CAD build for the part. Positions are in the model's coordinates, mm. Face numbers are marked on the shaded views. A direction names the side the tool comes from. Give positions to 0.01 mm unless a question says otherwise; leave off trailing zeros. Loops run counter-clockwise (first coordinate to the right, second up) from the corner with the lowest first, then second, coordinate; pieces in that order, holes last. Notation, with made-up numbers: (87.25, 28.25) -> (118.25, 28.25) arc R20 cw to (118.25, 47.25) -> close; hole circle Ø8 at (20, 20). An arc over 180 degrees is marked (long way). Use one line per item in the form item = value.
```python
from build123d import *

# Parameters (mm, degrees)
SKETCH_R        = 1.8
PAD_DEPTH       = 5
POCKET_DEPTH    = 2.3800001144
POCKET001_DEPTH = 1
SKETCH003_R     = 3
POCKET002_DEPTH = 3


with BuildPart() as part:
    # Sketch → Pad (new body)
    with BuildSketch(Plane.XY):
        with BuildLine():
            ThreePointArc((-7, -13.2664991614), (7.7459666924, -12.8452325787), (15, 0))
            Line((15, 30), (15, 0))
            ThreePointArc((15, 30), (7.7459666924, 42.8452325787), (-7, 43.2664991614))
            Line((-7, 43.2664991614), (-7, -13.2664991614))
        make_face()
        with Locations((0, 30)):
            Circle(SKETCH_R, mode=Mode.SUBTRACT)
        Circle(SKETCH_R, mode=Mode.SUBTRACT)
    extrude(amount=PAD_DEPTH)

    # Sketch001 → Pocket (cut)
    with BuildSketch(Plane.XY.offset(5)):
        with BuildLine():
            ThreePointArc((9.76, 30), (0, 39.76), (-9.76, 30))
            Line((-9.76, 30), (-9.76, 2.54016e-05))
            ThreePointArc((-9.76, 2.54016e-05), (-1.27008e-05, -9.76), (9.76, 0))
            Line((9.76, 30), (9.76, 0))
        make_face()
        with BuildLine():
            ThreePointArc((5, 30), (0, 35), (-5, 30))
            Line((-5, 30), (-5, 0))
            ThreePointArc((-5, 0), (0, -5), (5, 0))
            Line((5, 30), (5, 0))
        make_face(mode=Mode.SUBTRACT)
    extrude(amount=-POCKET_DEPTH, mode=Mode.SUBTRACT)

    # Sketch002 → Pocket001 (cut)
    with BuildSketch(Plane.XY.offset(5)):
        with BuildLine():
            ThreePointArc((15, 30), (0, 45), (-15, 30))
            Line((-15, 30), (-15, 3.614e-07))
            ThreePointArc((-15, 3.614e-07), (-1.807e-07, -15), (15, 0))
            Line((15, 30), (15, 0))
        make_face()
        with BuildLine():
            ThreePointArc((13, 30), (0, 43), (-13, 30))
            Line((-13, 30), (-13, 3.614e-07))
            ThreePointArc((-13, 3.614e-07), (-1.807e-07, -13), (13, 0))
            Line((13, 30), (13, 0))
        make_face(mode=Mode.SUBTRACT)
    extrude(amount=-POCKET001_DEPTH, mode=Mode.SUBTRACT)

    # Sketch003 → Pocket002 (cut)
    with BuildSketch(Plane(origin=(0, 0, 0), x_dir=(1, 0, 0), z_dir=(0, 0, -1))):
        with Locations((0, -30)):
            Circle(SKETCH003_R)
        Polygon((-3, -1.7320508076), (-3, 1.7320508076), (0, 3.4641016151), (3, 1.7320508076), (3, -1.7320508076), (0, -3.4641016151), align=None)
    extrude(amount=-POCKET002_DEPTH, mode=Mode.SUBTRACT)


solid = part.part
```
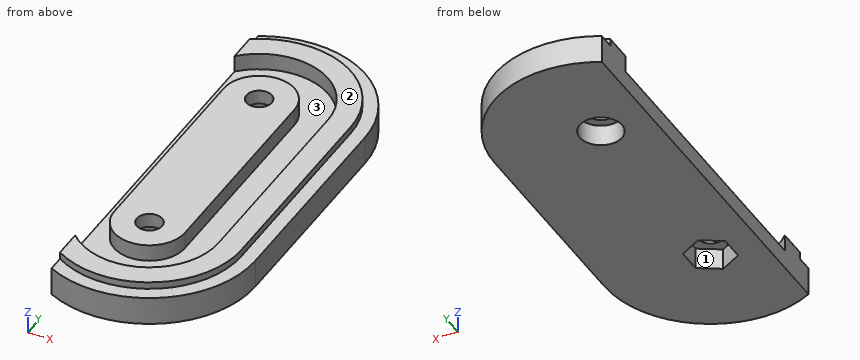
1. Drop flat-ended pins along their axis: P1, Ø1.8, axis at x = 0.5, y = 1, coming from the -Z side; P2, Ø6, axis at x = 0, y = 0, coming from the +Z side; P3, Ø1.2, axis at y = 15.5, z = 4, coming from the -X side; P4, Ø3, axis at x = 0, y = 30, coming from the +Z side (3 decimals). Give the stop position or say it passes through.
Result sheet:
P1 = 3
P2 = 5
P3 = -5
P4 = through
2. Cut at D-D, the plane y = 2.5. Write the cut outline in (x, z), then the cut area to 3 significant figures.
Result sheet:
outline = (-7, 0) -> (-1.67, 0) -> (-1.67, 3) -> (1.67, 3) -> (1.67, 0) -> (15, 0) -> (15, 4) -> (13, 4) -> (13, 5) -> (9.76, 5) -> (9.76, 2.62) -> (5, 2.62) -> (5, 5) -> (-5, 5) -> (-5, 2.62) -> (-7, 2.62) -> close
area = 81.9 mm^2
3. Cut at A-A, the plane z = 2.1. Write the cut outline in (x, y), then the cut area to 3 significant figures.
Result sheet:
outline = (-7, -13.27) arc R15 ccw to (15, 0) -> (15, 30) arc R15 ccw to (-7, 43.27) -> close; hole (-3, -1.73) -> (0, -3.46) -> (3, -1.73) -> (3, 1.73) -> (0, 3.46) -> (-3, 1.73) -> close; hole circle Ø6 at (0, 30)
area = 1,160 mm^2
4. Cut at C-C, the plane x = 11.5. Write the cut outline in (y, z), then the cut area to 3 significant figures.
Result sheet:
outline = (-9.63, 0) -> (39.63, 0) -> (39.63, 4) -> (36.06, 4) -> (36.06, 5) -> (-6.06, 5) -> (-6.06, 4) -> (-9.63, 4) -> close
area = 239 mm^2
5. Cut at B-B, the plane y = 18. Write the cut outline in (x, z).
Result sheet:
outline = (-7, 0) -> (15, 0) -> (15, 4) -> (13, 4) -> (13, 5) -> (9.76, 5) -> (9.76, 2.62) -> (5, 2.62) -> (5, 5) -> (-5, 5) -> (-5, 2.62) -> (-7, 2.62) -> close
6. Drill centre lines: line 1 (Y direction, x = 0, z = 1.8); line 2 (X direction, y = 0, z = 4.05); line 3 (Y direction, x = 0, z = 3.95). Where is each one in solid material? Low to high.
Result sheet:
line_1 = -15 to -3.46, 3.46 to 27, 33 to 45
line_2 = -5 to -1.8, 1.8 to 5, 9.76 to 13
line_3 = -15 to -9.76, -5 to -1.8, 1.8 to 28.2, 31.8 to 35, 39.76 to 45
7. Tool access for the marked faces 1, 2 and 3: list every direction of +Z, -Z, +X, -X, +Y, -Y with a clear straight run to the whole face (end or side of a thin tool).
Result sheet:
face_1 = -Z
face_2 = +Z, +X, -X, +Y, -Y
face_3 = +Z
